Model file for the job. Use its own axes, mm. A direction names the side the tool comes from. Coordinates: 2 decimals unless noted, no trailing zeros. Write each loop counter-clockwise with the first axis right and the second up, starting at its lowest first coordinate (ties: lowest second). Pieces come first, ordered by that corner, then holes. Notation, with made-up numbers: (60, 12.5) -> (102, 12.5) arc R22 cw to (102, 31.5) -> close; hole circle Ø9 at (75.25, 52). An arc over 180 degrees is marked (long way). Write item = value, one per line. Start each with the question number.
from build123d import *

# Parameters (mm, degrees)
SKETCH1_W           = 60
SKETCH1_H           = 26
BOSS_EXTRUDE2_DEPTH = 10
SKETCH1_5_W         = 56
SKETCH1_5_H         = 22
CUT_EXTRUDE1_DEPTH  = 6
CHAMFER1_SIZE       = 5
SKETCH2_W           = 14.5
SKETCH2_H           = 14.5
CUT_EXTRUDE2_DEPTH  = 34.241540277
CHAMFER2_SIZE       = 5
SKETCH3_W           = 18
SKETCH3_H           = 18
CUT_EXTRUDE3_DEPTH  = 1.5
SKETCH4_R           = 3
BOSS_EXTRUDE4_DEPTH = 1.5
SKETCH5_R           = 2
BOSS_EXTRUDE5_DEPTH = 1.175
SKETCH6_R           = 1.5
SKETCH6_R_2         = 0.875
BOSS_EXTRUDE6_DEPTH = 4.5
CHAMFER3_SIZE       = 2
FILLET1_R           = 3
CHAMFER4_SIZE       = 0.75
CHAMFER4_SIZE2      = 2.060608065


with BuildPart() as part:
    # Sketch1 → Boss-Extrude2 (new body)
    with BuildSketch(Plane.XY):
        Rectangle(SKETCH1_W, SKETCH1_H)
    extrude(amount=BOSS_EXTRUDE2_DEPTH)

    # Sketch1<5> → Cut-Extrude1 (cut)
    with BuildSketch(Plane.XY):
        Rectangle(SKETCH1_5_W, SKETCH1_5_H)
    extrude(amount=CUT_EXTRUDE1_DEPTH, mode=Mode.SUBTRACT)

    # Chamfer1
    chamfer1_edges = [part.edges().sort_by_distance(p)[0] for p in [
        (28, 11, 3),
        (-28, 11, 3),
        (-28, -11, 3),
        (28, -11, 3),
    ]]
    chamfer(chamfer1_edges, length=CHAMFER1_SIZE)

    # Sketch2 → Cut-Extrude2 (cut, through all)
    with BuildSketch(Plane(origin=(0, 0, 6), x_dir=(-1, 0, 0), z_dir=(0, 0, -1))):
        Rectangle(SKETCH2_W, SKETCH2_H)
    extrude(amount=-CUT_EXTRUDE2_DEPTH, mode=Mode.SUBTRACT)

    # Chamfer2
    chamfer2_edges = [part.edges().sort_by_distance(p)[0] for p in [
        (30, 13, 5),
        (30, -13, 5),
        (-30, -13, 5),
        (-30, 13, 5),
    ]]
    chamfer(chamfer2_edges, length=CHAMFER2_SIZE)

    # Sketch3 → Cut-Extrude3 (cut)
    with BuildSketch(Plane.XY.offset(10)):
        Polygon((-28.5, 7.378679656), (-28.5, -7.378679656), (-24.378679656, -11.5), (24.378679656, -11.5), (28.5, -7.378679656), (28.5, 7.378679656), (24.378679656, 11.5), (-24.378679656, 11.5), align=None)
        Rectangle(SKETCH3_W, SKETCH3_H, mode=Mode.SUBTRACT)
    extrude(amount=-CUT_EXTRUDE3_DEPTH, mode=Mode.SUBTRACT)

    # Sketch4 → Boss-Extrude4 (add)
    with BuildSketch(Plane.XY.offset(8.5)):
        with Locations((-20.5, 0)):
            Circle(SKETCH4_R)
    boss_extrude4 = extrude(amount=BOSS_EXTRUDE4_DEPTH)

    # Sketch5 → Boss-Extrude5 (add)
    with BuildSketch(Plane.XY.offset(10)):
        with Locations((-20.5, 0)):
            Circle(SKETCH5_R)
    boss_extrude5 = extrude(amount=BOSS_EXTRUDE5_DEPTH)

    # Mirror1: Boss-Extrude4, Boss-Extrude5 across plane
    add(boss_extrude4.mirror(Plane(origin=(0, 0, 0), x_dir=(0, 0, 1), z_dir=(1, 0, 0))))
    add(boss_extrude5.mirror(Plane(origin=(0, 0, 0), x_dir=(0, 0, 1), z_dir=(1, 0, 0))))

    # Sketch6 → Boss-Extrude6 (add)
    # profile 1 of 2: a face of its own
    with BuildSketch(Plane(origin=(0, 0, 6), x_dir=(-1, 0, 0), z_dir=(0, 0, -1))):
        with Locations(Location((-18.891430022, -8.28, 0), (0, 0, 180))):
            Circle(SKETCH6_R)
        with Locations((-18.891430022, -8.28)):
            Circle(SKETCH6_R_2, mode=Mode.SUBTRACT)
    # profile 2 of 2: a face of its own
    with BuildSketch(Plane(origin=(0, 0, 6), x_dir=(-1, 0, 0), z_dir=(0, 0, -1))):
        with Locations(Location((20.972750365, 8.32, 0), (0, 0, 180))):
            Circle(SKETCH6_R)
        with Locations((20.972750365, 8.32)):
            Circle(SKETCH6_R_2, mode=Mode.SUBTRACT)
    extrude(amount=BOSS_EXTRUDE6_DEPTH)

    # Chamfer3
    # the kernel refuses this chamfer: 2 mm, written as the material it adds along each edge
    with BuildSketch(Plane(origin=(18.891430022, -8.28, 6), x_dir=(1, 0, 0), z_dir=(0, 1, 0))) as chamfer3_piece_1:
        Polygon((1.5 + CHAMFER3_SIZE, 0), (1.5, CHAMFER3_SIZE), (1.5, 0), align=None)
    revolve(axis=Axis((18.891430022, -8.28, 6), (0, 0, -1)))
    with BuildSketch(Plane(origin=(-20.972750365, 8.32, 6), x_dir=(1, 0, 0), z_dir=(0, 1, 0))) as chamfer3_piece_2:
        Polygon((1.5 + CHAMFER3_SIZE, 0), (1.5, CHAMFER3_SIZE), (1.5, 0), align=None)
    revolve(axis=Axis((-20.972750365, 8.32, 6), (0, 0, -1)))

    # Fillet1
    fillet1_edges = [part.edges().sort_by_distance(p)[0] for p in [
        (25, -13, 5),
        (-25, -13, 5),
        (-30, 8, 5),
        (-30, -8, 5),
        (30, 8, 5),
        (30, -8, 5),
        (-25, 13, 5),
        (25, 13, 5),
    ]]
    fillet(fillet1_edges, radius=FILLET1_R)

    # Chamfer4
    chamfer4_edges = [part.edges().sort_by_distance(p)[0] for p in [
        (30, 0, 10),
        (-30, 0, 10),
        (-27.5, -10.5, 10),
        (0, -13, 10),
        (27.5, -10.5, 10),
        (27.5, 10.5, 10),
        (0, 13, 10),
        (-27.5, 10.5, 10),
        (29.771638598, -7.90540961, 10),
        (24.90540961, -12.771638598, 10),
        (-24.90540961, -12.771638598, 10),
        (-29.771638598, -7.90540961, 10),
        (-29.771638598, 7.90540961, 10),
        (-24.90540961, 12.771638598, 10),
        (24.90540961, 12.771638598, 10),
        (29.771638598, 7.90540961, 10),
    ]]
    chamfer4_side = [part.faces().sort_by_distance(p)[0] for p in [
        (-29.346088691, 0, 10),
    ]]
    chamfer(chamfer4_edges, length=CHAMFER4_SIZE, length2=CHAMFER4_SIZE2, reference=chamfer4_side[0])


solid = part.part
(1) Drop flat-ended pins along their axis: pin 1 Ø1.2 at (x, z) = (-1, 9.5) entering from +Y; pin 2 Ø3 at (x, z) = (-3.5, 8) entering from -Y; pin 3 Ø1 at (y, z) = (-9.5, 1.5) entering from -X; pin 4 Ø2 at (y, z) = (10.5, 8.5) entering from +X. Give the stop position or say it passes through.
(2) Mould opens along X. For faces 1 (the face through (0, 13, 4)), 2 (the face through (-20.278, 7.788, 3.782)), 3 (the face through (-24.921, -12.765, 4.025)) say: released by +X, released by -X, zero draft, split by the parting line, or undercut.
(3) Saw through at B-B (x = 10). Give the cut face in (y, z).
(4) Drill centre lines: line 1 along X through (y, z) = (-1.5, 1.25); line 2 along Y through (x, z) = (5, 3.75); line 3 along X through (y, z) = (10.25, 4.75). Where is each one in solid material? Low to high.
(5) 3-axis set-ups, long thin cutter, end or side, ignore diameter. For faces 4 (the face through (-20, 9, 1.5)), 5 (the face through (-7.25, 0, 8)), 6 (the face through (-9, 0, 9)), 7 (the face through (-8, 0, 10)), 8 (the face through (21, 0, 11.175)): which of +Z, -Z, +X, -X, +Y, -Y reach the whole face in a straight line?
(6) Saw through at A-A (x = -5.5). Give the cut face in (y, z), then the cut area to 3 significant figures.
Returned:
q1.pin_1 = 12.65
q1.pin_2 = -13
q1.pin_3 = -29
q1.pin_4 = 28.34
q2.face_1 = zero draft
q2.face_2 = undercut
q2.face_3 = released by -X
q3.outline = (-13, 0) -> (-11, 0) -> (-11, 6) -> (11, 6) -> (11, 0) -> (13, 0) -> (13, 7.94) -> (12.25, 10) -> (11.5, 10) -> (11.5, 8.5) -> (-11.5, 8.5) -> (-11.5, 10) -> (-12.25, 10) -> (-13, 7.94) -> close
q4.line_1 = -30 to -28, 28 to 30
q4.line_2 = -13 to -11, 11 to 13
q4.line_3 = -27.75 to -23.75, -22.13 to -19.82, 23.75 to 27.75
q5.face_4 = -Z
q5.face_5 = +Z, -Z
q5.face_6 = +Z
q5.face_7 = +Z, +Y, -Y
q5.face_8 = +Z, +X, -X, +Y, -Y
q6.outline = (-13, 0) -> (-11, 0) -> (-11, 6) -> (-7.25, 6) -> (-7.25, 10) -> (-9, 10) -> (-9, 8.5) -> (-11.5, 8.5) -> (-11.5, 10) -> (-12.25, 10) -> (-13, 7.94) -> close; (7.25, 6) -> (11, 6) -> (11, 0) -> (13, 0) -> (13, 7.94) -> (12.25, 10) -> (11.5, 10) -> (11.5, 8.5) -> (9, 8.5) -> (9, 10) -> (7.25, 10) -> close
q6.area = 61.0 mm2
